Job drawing, mm, ordinate dimensions from the low corner. One solid piece. Give positions to 0.01 mm unless a question says otherwise; leave off trailing zeros. Write each loop counter-clockwise with the first axis right and the second up, starting at its lowest first coordinate (ties: lowest second). Pieces come first, ordered by that corner, then holes. Notation, with made-up numbers: (-37, 88.25) - (-30, 88.25) arc R17 cw to (-30, 115.25) - close; hole circle Ø11 at (14, 4.25). An arc over 180 degrees is marked (long way). Put each result on its own line as item: value. Start each with the question number.
1. Cut at A-A on x = 32. List the corners of the cut face in (y, z).
2. Cut at C-C on y = 5.5. List the corners of the cut face in (x, z), and give its area (3 significant figures).
3. Wall check: line 1 (Z direction, x = 56.5, y = 18.5); line 2 (Z direction, x = 33, y = 5). Give the ranges that are in metal, low to high.
4. Cut at B-B on y = 44.5. List the corners of the cut face in (x, z).
5. Drop flat-ended pins along their axis: pin 1 (4 mm diameter, centred on x = 29, z = 264.5, fed in from -Y); pin 2 (1.5 mm diameter, centred on x = 45, y = 38.5, fed in from -Z); pin 3 (1 mm diameter, centred on x = 63, y = 18.5, fed in from -Z). Give the stop position or say it passes through.
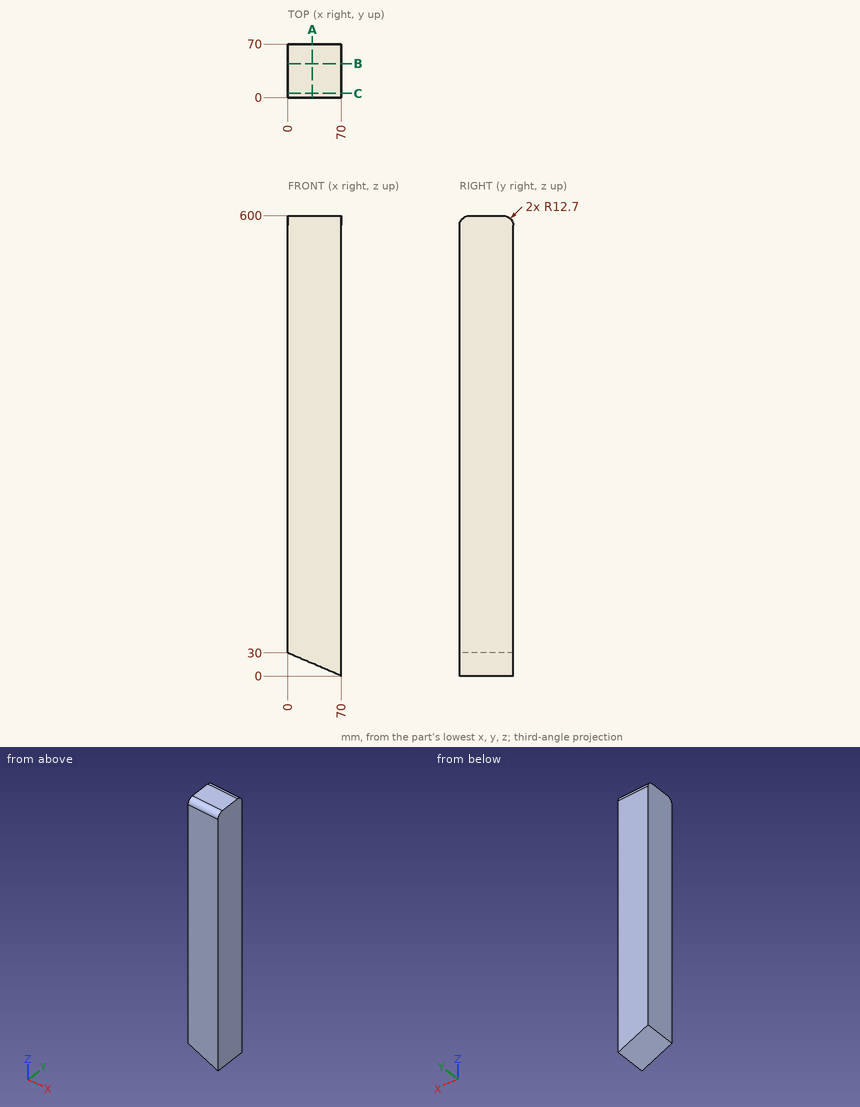
Report:
1. outline: (0, 16.29) - (70, 16.29) - (70, 587.3) arc R12.7 ccw to (57.3, 600) - (12.7, 600) arc R12.7 ccw to (0, 587.3) - close
2. outline: (0, 30) - (70, 0) - (70, 597.76) - (0, 597.76) - close
2. area: 40,800 mm²
3. line 1: z = 5.79 to 600
3. line 2: z = 15.86 to 597.4
4. outline: (0, 30) - (70, 0) - (70, 600) - (0, 600) - close
5. pin 1: stops at y = 0
5. pin 2: stops at z = 10.39
5. pin 3: stops at z = 2.79
